from build123d import *

# Parameters (mm, degrees)
ESQUISSE1_R             = 9.5
BASE_EXTRUSION_DEPTH    = 17
ESQUISSE2_R             = 8.5
ENL_V_MAT_EXTRU_1_DEPTH = 5.5
ESQUISSE3_R             = 2
ENL_V_MAT_EXTRU_2_DEPTH = 15
ENL_V_MAT_EXTRU_3_DEPTH = 10
CONG_1_R                = 1


with BuildPart() as part:
    # Esquisse1 → Base-Extrusion (new body)
    with BuildSketch(Plane.XY):
        Circle(ESQUISSE1_R)
    extrude(amount=BASE_EXTRUSION_DEPTH)

    # Esquisse2 → Enlèv. mat.-Extru.1 (cut)
    with BuildSketch(Plane.XY.offset(17)):
        Circle(ESQUISSE2_R)
    extrude(amount=-ENL_V_MAT_EXTRU_1_DEPTH, mode=Mode.SUBTRACT)

    # Esquisse3 → Enlèv. mat.-Extru.2 (cut, symmetric)
    with BuildSketch(Plane(origin=(0, 0, 0), x_dir=(1, 0, 0), z_dir=(0, 1, 0))):
        with Locations(Location((0, -7.5, 0), (0, 0, 270))):
            Circle(ESQUISSE3_R)
        with BuildLine():
            Line((-5, -17), (5, -17))
            Line((5, -17), (5, -15))
            ThreePointArc((5, -15), (4.414213562, -13.585786438), (3, -13))
            Line((3, -13), (-3, -13))
            ThreePointArc((-3, -13), (-4.414213562, -13.585786438), (-5, -15))
            Line((-5, -15), (-5, -17))
        make_face()
    extrude(amount=ENL_V_MAT_EXTRU_2_DEPTH, both=True, mode=Mode.SUBTRACT)

    # Esquisse4 → Enlèv. mat.-Extru.3 (cut)
    with BuildSketch(Plane.XY.offset(11.5)):
        with BuildLine():
            Line((-4.769696007, 3.5), (4.769696007, 3.5))
            ThreePointArc((4.769696007, 3.5), (5.952911964, 3.11245155), (6.67757441, 2.1))
            ThreePointArc((6.67757441, 2.1), (7, 0), (6.67757441, -2.1))
            ThreePointArc((6.67757441, -2.1), (5.952911964, -3.11245155), (4.769696007, -3.5))
            Line((4.769696007, -3.5), (-4.769696007, -3.5))
            ThreePointArc((-4.769696007, -3.5), (-5.952911964, -3.11245155), (-6.67757441, -2.1))
            ThreePointArc((-6.67757441, -2.1), (-7, 0), (-6.67757441, 2.1))
            ThreePointArc((-6.67757441, 2.1), (-5.952911964, 3.11245155), (-4.769696007, 3.5))
        make_face()
    extrude(amount=-ENL_V_MAT_EXTRU_3_DEPTH, mode=Mode.SUBTRACT)

    # Congé1
    cong_1_edges = [part.edges().sort_by_distance(p)[0] for p in [
        (0, 3.5, 1.5),
        (0, -3.5, 1.5),
        (-5.952911964, 3.11245155, 1.5),
        (5.952911964, 3.11245155, 1.5),
        (7, 0, 1.5),
        (5.952911964, -3.11245155, 1.5),
        (-5.952911964, -3.11245155, 1.5),
        (-7, 0, 1.5),
    ]]
    fillet(cong_1_edges, radius=CONG_1_R)


solid = part.part
Part model, mm, in its own coordinate system. A direction names the side the tool comes from. Give positions to 0.01 mm unless a question says otherwise; leave off trailing zeros. Loops run counter-clockwise (first coordinate to the right, second up) from the corner with the lowest first, then second, coordinate; pieces in that order, holes last. Notation, with made-up numbers: (85.25, 28) -> (98.25, 28) arc R15 cw to (98.25, 43) -> close; hole circle Ø7 at (55, 14.5). An arc over 180 degrees is marked (long way). Write each question's results on one line, items separated by ' | '. Start each with the question number.
Q1. Band-saw the part on C-C on z = 7.5. List the corners of the cut face in (x, y), plus the area to 3 significant figures.
Q2. Wall check: L1, parallel to X at y = 5, z = 7.5; L2, parallel to X at y = 6.75, z = 7.5; L3, parallel to Z at x = 0, y = 5.5. Give the ranges that are in metal, low to high.
Q3. Pull direction Y, two halves, no side cores. Call faces 4 (the face through (-0.067, -3.215, 1.801)), 5 (the face through (0.088, 6.545, 5.502)): +Y half, -Y half, draft (parallel to the pull), parting line (faces both ways), or undercut.
Q4. Which spindle directions (+Z, -Z, +X, -X, +Y, -Y) get a long thin tool onto all of the face, cutting with end or side? Do faces 1 (the face through (4.43, -7.93, 13.6)), 2 (the face through (9, 0, 17)), 3 (the face through (-8.49, 0.37, 13.68)). Say none if no direction does.
Q5. Band-saw the part on A-A on x = 0. List the corners of the cut face in (y, z), plus the area to 3 significant figures.
Q6. Pin check, flat tips, straight feed: P1, Ø5, axis at x = -5.5, z = 10.5, coming from the -Y side; P2, Ø1, axis at x = -7, z = 14, coming from the -Y side; P3, Ø2.5, axis at x = -2.5, y = -0.5, coming from the +Z side; P4, Ø4.5, axis at x = 0, z = 7.5, coming from the +Y side. Stop position of each tip, or through.
Q7. Band-saw the part on B-B on y = 0. List the corners of the cut face in (x, z), plus the area to 3 significant figures.
Q8. Band-saw the part on D-D on y = 4.25. List the corners of the cut face in (x, z), plus the area to 3 significant figures.
Results are:
1) outline: (-6.68, -2.1) arc R7 cw to (-6.68, 2.1) arc R2 cw to (-4.77, 3.5) -> (-2, 3.5) -> (-2, 9.29) arc R9.5 ccw to (-2, -9.29) -> (-2, -3.5) -> (-4.77, -3.5) arc R2 cw to start; (2, -9.29) arc R9.5 ccw to (2, 9.29) -> (2, 3.5) -> (4.77, 3.5) arc R2 cw to (6.68, 2.1) arc R7 cw to (6.68, -2.1) arc R2 cw to (4.77, -3.5) -> (2, -3.5) -> close | area: 144 mm²
2) L1: x = -8.08 to -2, 2 to 8.08 | L2: x = -6.68 to -2, 2 to 6.68 | L3: z = 0 to 5.5, 9.5 to 11.5
3) face 4: undercut | face 5: draft
4) face 1: +Z, +Y, -Y | face 2: +Z, +X, -X, +Y, -Y | face 3: +Z
5) outline: (-9.5, 0) -> (9.5, 0) -> (9.5, 5.5) -> (3.5, 5.5) -> (3.5, 2.5) arc R1 cw to (2.5, 1.5) -> (-2.5, 1.5) arc R1 cw to (-3.5, 2.5) -> (-3.5, 5.5) -> (-9.5, 5.5) -> close; (-9.5, 9.5) -> (-3.5, 9.5) -> (-3.5, 11.5) -> (-8.5, 11.5) -> (-8.5, 13) -> (-9.5, 13) -> close; (3.5, 9.5) -> (9.5, 9.5) -> (9.5, 13) -> (8.5, 13) -> (8.5, 11.5) -> (3.5, 11.5) -> close | area: 104 mm²
6) P1: stops at y = -9.01 | P2: stops at y = -6.93 | P3: stops at z = 1.5 | P4: stops at y = 9.5
7) outline: (-9.5, 0) -> (9.5, 0) -> (9.5, 17) -> (8.5, 17) -> (8.5, 11.5) -> (7, 11.5) -> (7, 2.5) arc R1 cw to (6, 1.5) -> (-6, 1.5) arc R1 cw to (-7, 2.5) -> (-7, 11.5) -> (-8.5, 11.5) -> (-8.5, 17) -> (-9.5, 17) -> close | area: 89.9 mm²
8) outline: (-8.5, 0) -> (8.5, 0) -> (8.5, 17) -> (7.36, 17) -> (7.36, 11.5) -> (-7.36, 11.5) -> (-7.36, 17) -> (-8.5, 17) -> close; hole circle Ø4 at (0, 7.5) | area: 195 mm²
